Build history of the part. All positions in model axes, mm. A direction names the side the tool comes from. Give positions to 0.01 mm unless a question says otherwise; leave off trailing zeros. Write each loop counter-clockwise with the first axis right and the second up, starting at its lowest first coordinate (ties: lowest second). Pieces come first, ordered by that corner, then holes.
Autodesk Inventor part; units mm, degrees
ref_plane "YZ Plane" through (0, 0, 0) normal (1, 0, 0) x (0, 1, 0)
ref_plane "XZ Plane" through (0, 0, 0) normal (0, 1, 0) x (-1, 0, 0)
ref_plane "XY Plane" through (0, 0, 0) normal (0, 0, 1) x (1, 0, 0)
sketch "Sketch1" plane through (0, 0, 0) normal (0, 0, 1) x (1, 0, 0)
  line L0 (0, 6) -> (0, 8)
  line L1 (0, 8) -> (12, 8)
  line L2 (12, 8) -> (12, 4)
  line L3 (12, 4) -> (0, 4)
  line L4 (0, 6) -> (0, 4)
  point P0 (0, 0)
  dimension "d2" = 2
  dimension "d3" = 4
extrude "Extrusion1" add sketch "Sketch1" along normal blind 5
sketch "Sketch2" plane through (0, 0, 5) normal (0, 0, 1) x (1, 0, 0)
  line L0 (0, 8) -> (0, 4)
  line L1 (12, 4) -> (12, 8)
  line L2 (12, 8) -> (0, 8)
  line L3 (0, 4) -> (12, 4)
  line L4 (0, 6) -> (12, 6)
  line L5 (6, 8) -> (6, 4)
  circle A0 centre (6, 6) radius 5
  point P0 (0, 0)
  dimension "d9" = 10
extrude "Extrusion3" add sketch "Sketch2" along normal blind 1 contours A0 L2 | L2 L5 L4 A0 | L4 L5 L3 A0 | L2 A0 L4 L5 | L3 A0 | L4 A0 L3 L5
properties part number "MinusBtn"
1. Drill centre lines: line 1 along Y through (x, z) = (2.5, 4.5); line 2 along Z through (x, y) = (9, 8.5); line 3 along Z through (x, y) = (11, 7). Where is each one in solid material? Low to high.
2. Saw through at D-D on y = 9. Give the cut face in (x, z), plus the area to 3 significant figures.
3. Saw through at A-A on x = 6. Give the cut face in (y, z), plus the area to 3 significant figures.
4. Drop flat-ended pins along their axis: pin 1 (0.7 mm diameter, centred on x = 0.5, y = 6, fed in from +Z); pin 2 (0.9 mm diameter, centred on x = 5.5, y = 10, fed in from -Z); pin 3 (2.5 mm diameter, centred on x = 5.5, z = 2.5, fed in from -Y). Give the stop position or say it passes through.
5. 3-axis set-ups, long thin cutter, end or side, ignore diameter. For faces 1 (the face through (2, 9, 5.5)), 2 (the face through (6, 3, 5)), 3 (the face through (0, 6, 2)), 4 (the face through (6, 8, 2)), 5 (the face through (6, 6, 0)): which of +Z, -Z, +X, -X, +Y, -Y reach the whole face in a straight line?
6. Saw through at B-B on y = 6. Give the cut face in (x, z), plus the area to 3 significant figures.
7. Saw through at C-C on z = 4.8. Give the cut face in (x, y).
Outcome:
1. line 1: y = 4 to 8
1. line 2: z = 5 to 6
1. line 3: z = 0 to 5
2. outline: (2, 5) - (10, 5) - (10, 6) - (2, 6) - close
2. area: 8.00 mm2
3. outline: (1, 5) - (4, 5) - (4, 0) - (8, 0) - (8, 5) - (11, 5) - (11, 6) - (1, 6) - close
3. area: 30.0 mm2
4. pin 1: stops at z = 5
4. pin 2: stops at z = 5
4. pin 3: stops at y = 4
5. face 1: +Z
5. face 2: -Z, +X, -X, -Y
5. face 3: +Z, -Z, -X, +Y, -Y
5. face 4: -Z, +X, -X, +Y
5. face 5: -Z, +X, -X, +Y, -Y
6. outline: (0, 0) - (12, 0) - (12, 5) - (11, 5) - (11, 6) - (1, 6) - (1, 5) - (0, 5) - close
6. area: 70.0 mm2
7. outline: (0, 4) - (12, 4) - (12, 8) - (0, 8) - close
